Build history of the part. All positions in model axes, mm. Round coordinates to 2 decimals unless told otherwise and drop trailing zeros. Write each loop counter-clockwise with the first axis right and the second up, starting at its lowest first coordinate (ties: lowest second). Pieces come first, ordered by that corner, then holes. Notation, with made-up numbers: (-34.5, -26.5) - (17.5, -26.5) arc R31 cw to (17.5, 6.5) - close; hole circle Ø9 at (-24.5, -2). An arc over 180 degrees is marked (long way). One line per question, with ' | ' between items.
from build123d import *

# Parameters (mm, degrees)
S01_TPU_BEAD_AND_BEARING_OUTER_RACE_KE_R       = 34.9
S01_TPU_BEAD_AND_BEARING_OUTER_RACE_KE_R_2     = 24.8
F_01_TPU_BEAD_AND_BEARING_OUTER_RACE_KEE_DEPTH = 2.5
F_02_START                                     = -0.1
S02_FLANGE_SCREW_CLEARANCE_R                   = 1.7
F_02_FLANGE_SCREW_CLEARANCE_DEPTH              = 2.7


with BuildPart() as part:
    # S01 - TPU bead and bearing outer-race keeper → 01 - TPU bead and bearing outer-race keeper (new body)
    with BuildSketch(Plane.XY):
        Circle(S01_TPU_BEAD_AND_BEARING_OUTER_RACE_KE_R)
        Circle(S01_TPU_BEAD_AND_BEARING_OUTER_RACE_KE_R_2, mode=Mode.SUBTRACT)
    extrude(amount=F_01_TPU_BEAD_AND_BEARING_OUTER_RACE_KEE_DEPTH)

    # S02 - Flange screw clearance → 02 - Flange screw clearance (cut)
    with BuildSketch(Plane.XY.offset(F_02_START)):
        with Locations(Location((28.832885915, 7.725748496, 0), (0, 0, 180))):
            Circle(S02_FLANGE_SCREW_CLEARANCE_R)
        with Locations(Location((-21.107137418, 21.107137418, 0), (0, 0, 180))):
            Circle(S02_FLANGE_SCREW_CLEARANCE_R)
        with Locations(Location((-7.725748496, -28.832885915, 0), (0, 0, 180))):
            Circle(S02_FLANGE_SCREW_CLEARANCE_R)
    extrude(amount=F_02_FLANGE_SCREW_CLEARANCE_DEPTH, mode=Mode.SUBTRACT)


solid = part.part
Q1. Drop flat-ended pins along their axis: pin 1 (1.5 mm diameter, centred on y = -3, z = 1, fed in from +X); pin 2 (1.5 mm diameter, centred on x = 13, z = 1.5, fed in from -Y); pin 3 (2.5 mm diameter, centred on x = 28.83, y = 7.73, fed in from +Z). Give the stop position or say it passes through.
Found:
pin 1: x = 34.83 | pin 2: y = -32.68 | pin 3: through
Q2. Drill centre lines: L1, parallel to Y at x = 0, z = 1.35; L2, parallel to X at y = 8.5, z = 0.7; L3, parallel to X at y = 20, z = 1.6. Where is each one in solid material? Low to high. Write a range as from..to.
Found:
L1: -34.9..-24.8, 24.8..34.9 | L2: -33.85..-23.3, 23.3..27.32, 30.35..33.85 | L3: -28.6..-22.4, -19.82..-14.66, 14.66..28.6
Q3. Saw through at C-C, the plane z = 1.15. List the corners of the cut face in (x, y), then the cut area to 3 significant figures.
Found:
outline: circle Ø69.8 at (0, 0); hole circle Ø49.6 at (0, 0); hole circle Ø3.4 at (-21.11, 21.11); hole circle Ø3.4 at (-7.73, -28.83); hole circle Ø3.4 at (28.83, 7.73) | area: 1,870 mm^2
Q4. Pull direction X, two halves, no side cores. Call faces 1 (the cylindrical face through (-7.57, -34.07, 1.23)), 2 (the cylindrical face through (-7.357, -27.173, 1.232)), 3 (the cylindrical face through (30.53, 7.65, 1.23)), 4 (the flat face through (-24, -7, 0)): +X half, -X half, draft (parallel to the pull), parting line (faces both ways), or undercut.
Found:
face 1: parting line | face 2: undercut | face 3: undercut | face 4: draft
Q5. Saw through at D-D, the plane y = 26. List the corners of the cut face in (x, z), then the cut area to 3 significant figures.
Found:
outline: (-23.28, 0) - (23.28, 0) - (23.28, 2.5) - (-23.28, 2.5) - close | area: 116 mm^2
Q6. Saw through at A-A, the plane y = 0. List the corners of the cut face in (x, z).
Found:
outline: (-34.9, 0) - (-24.8, 0) - (-24.8, 2.5) - (-34.9, 2.5) - close; (24.8, 0) - (34.9, 0) - (34.9, 2.5) - (24.8, 2.5) - close
